Part print with two shaded views. Sizes in mm from the minimum x, y, z corner. A direction names the side the tool comes from. Coordinates: 2 decimals unless noted, no trailing zeros. Write each loop counter-clockwise with the first axis right and the second up, starting at its lowest first coordinate (ties: lowest second). Pieces come first, ordered by that corner, then holes.
Q1. Band-saw the part on C-C, the plane y = 420. Write the cut outline in (x, z).
Q2. Pin check, flat tips, straight feed: P1, Ø4, axis at x = 167.5, z = 33, coming from the +Y side; P2, Ø24, axis at x = 200.5, z = 51.5, coming from the -Y side; P3, Ø1.5, axis at y = 68, z = 66.5, coming from the -X side. Stop position of each tip, or through.
Q3. Which spindle directions (+Z, -Z, +X, -X, +Y, -Y) get a long thin tool onto all of the face, cutting with end or side? Do the marked faces 1, 2, 3, 4 and 5. Say none if no direction does.
Q4. Drill centre lines: probe 1 along X at (y, z) = (87, 29.5); probe 2 along Y at (x, z) = (88, 27.5). Where is each one in solid material? Low to high.
Q5. Band-saw the part on A-A, the plane x = 258. Write the cut outline in (y, z).
Q6. Band-saw the part on B-B, the plane z = 13.5. Write the cut outline in (x, y), plus the area to 3 significant figures.
Q7. Pull direction X, two halves, no side cores. Call the marked faces 6, 7, 8 and 9: released by +X, released by -X, zero draft, split by the parting line, or undercut.
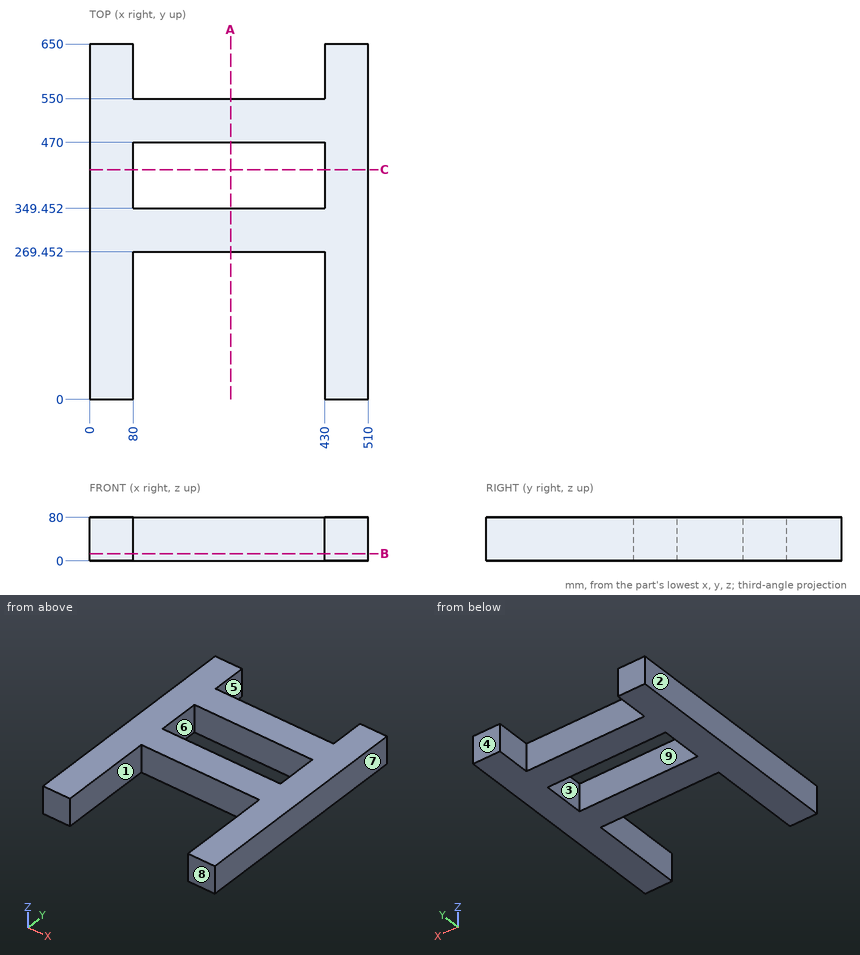
Answer sheet:
1. outline: (0, 0) - (80, 0) - (80, 80) - (0, 80) - close; (430, 0) - (510, 0) - (510, 80) - (430, 80) - close
2. P1: stops at y = 550
2. P2: stops at y = 269.45
2. P3: stops at x = 0
3. face 1: +Z, -Z, -Y
3. face 2: +Z, -Z, -X, +Y, -Y
3. face 3: +Z, -Z
3. face 4: +Z, -Z, +X, -X, +Y
3. face 5: +Z, -Z, +Y
4. probe 1: x = 0 to 80, 430 to 510
4. probe 2: y = 269.45 to 349.45, 470 to 550
5. outline: (269.45, 0) - (349.45, 0) - (349.45, 80) - (269.45, 80) - close; (470, 0) - (550, 0) - (550, 80) - (470, 80) - close
6. outline: (0, 0) - (80, 0) - (80, 269.45) - (430, 269.45) - (430, 0) - (510, 0) - (510, 650) - (430, 650) - (430, 550) - (80, 550) - (80, 650) - (0, 650) - close; hole (80, 349.45) - (430, 349.45) - (430, 470) - (80, 470) - close
6. area: 160,000 mm2
7. face 6: undercut
7. face 7: released by +X
7. face 8: zero draft
7. face 9: undercut
